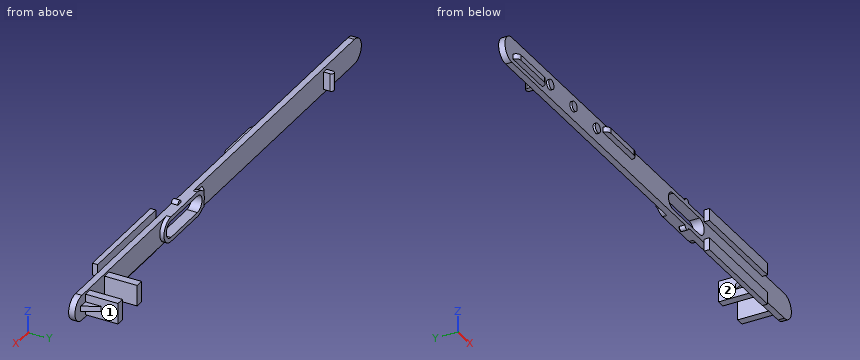
from build123d import *

# Parameters (mm, degrees)
BOSS_EXTRUDE1_DEPTH  = 1.2
BOSS_EXTRUDE2_DEPTH  = 0.8
SKETCH3_W            = 20
SKETCH3_H            = 2.3
BOSS_EXTRUDE3_DEPTH  = 1
SKETCH4_W            = 20
SKETCH4_H            = 2.3
BOSS_EXTRUDE4_DEPTH  = 1
CUT_EXTRUDE1_START   = -0.8
CUT_EXTRUDE1_DEPTH   = 0.8
CUT_EXTRUDE2_START   = -0.8
CUT_EXTRUDE2_DEPTH   = 0.8
CUT_EXTRUDE3_DEPTH   = 50.502424183
BOSS_EXTRUDE5_DEPTH  = 1.2
BOSS_EXTRUDE6_DEPTH  = 1.2
SKETCH10_W           = 1.5
SKETCH10_H           = 4
BOSS_EXTRUDE7_DEPTH  = 6.2
SKETCH11_W           = 1.5
SKETCH11_H           = 4
BOSS_EXTRUDE8_DEPTH  = 6.2
BOSS_EXTRUDE9_DEPTH  = 3.4
BOSS_EXTRUDE10_DEPTH = 1
BOSS_EXTRUDE11_DEPTH = 1
DRAFT1_ANGLE         = 45
SKETCH15_W           = 0.9
SKETCH15_H           = 0.4
SKETCH16_W           = 0.9
SKETCH16_H           = 0.4
SKETCH17_W           = 0.9
SKETCH17_H           = 0.4
RIB1_REACH           = 52.012
SKETCH18_WALL_W      = 105.424996876
SKETCH18_WALL_H      = 1
RIB2_REACH           = 52.012
SKETCH19_WALL_W      = 105.424996876
SKETCH19_WALL_H      = 1
FILLET2_R            = 0.1


with BuildPart() as part:
    # Sketch1 → Boss-Extrude1 (new body)
    with BuildSketch(Plane.XZ):
        with BuildLine():
            Line((46.9, 2.4), (-46.9, 2.4))
            ThreePointArc((-46.9, 2.4), (-49.3, 0), (-46.9, -2.4))
            Line((-46.9, -2.4), (46.9, -2.4))
            ThreePointArc((46.9, -2.4), (49.3, 0), (46.9, 2.4))
        make_face()
    extrude(amount=-BOSS_EXTRUDE1_DEPTH)

    # Sketch2 → Boss-Extrude2 (add)
    with BuildSketch(Plane(origin=(0, 1.2, 0), x_dir=(-1, 0, 0), z_dir=(0, 1, 0))):
        with BuildLine():
            Line((-6.33, 2.4), (-6.33, 0.918))
            Line((-6.33, 0.918), (-6.382506821, 0.918))
            ThreePointArc((-6.382506821, 0.918), (-6.2, 0), (-6.382506821, -0.918))
            Line((-6.382506821, -0.918), (-6.33, -0.918))
            Line((-6.33, -0.918), (-6.33, -2.4))
            Line((-6.33, -2.4), (-17.7, -2.4))
            ThreePointArc((-17.7, -2.4), (-20.1, 0), (-17.7, 2.4))
            Line((-17.7, 2.4), (-6.33, 2.4))
        make_face()
    extrude(amount=BOSS_EXTRUDE2_DEPTH)

    # Sketch3 → Boss-Extrude3 (add)
    with BuildSketch(Plane.XZ):
        with Locations((29.3, 2.85)):
            Rectangle(SKETCH3_W, SKETCH3_H)
    extrude(amount=BOSS_EXTRUDE3_DEPTH)

    # Sketch4 → Boss-Extrude4 (add)
    with BuildSketch(Plane.XZ):
        with Locations((29.3, -2.85)):
            Rectangle(SKETCH4_W, SKETCH4_H)
    extrude(amount=BOSS_EXTRUDE4_DEPTH)

    # Sketch5 → Cut-Extrude1 (cut)
    with BuildSketch(Plane(origin=(0, 2, 0), x_dir=(-1, 0, 0), z_dir=(0, 1, 0)).offset(CUT_EXTRUDE1_START)):
        with BuildLine():
            Line((-8.6, -2.4), (-6.33, -2.4))
            Line((-6.33, -2.4), (-6.33, -1.697))
            Line((-6.33, -1.697), (-6.902887452, -1.697))
            ThreePointArc((-6.902887452, -1.697), (-7.681523, -2.21729565), (-8.6, -2.4))
        make_face()
    extrude(amount=CUT_EXTRUDE1_DEPTH, mode=Mode.SUBTRACT)

    # Sketch6 → Cut-Extrude2 (cut)
    with BuildSketch(Plane(origin=(0, 2, 0), x_dir=(-1, 0, 0), z_dir=(0, 1, 0)).offset(CUT_EXTRUDE2_START)):
        with BuildLine():
            Line((-6.902887452, 1.697), (-6.33, 1.697))
            Line((-6.33, 1.697), (-6.33, 2.4))
            Line((-6.33, 2.4), (-8.6, 2.4))
            ThreePointArc((-8.6, 2.4), (-7.681523, 2.21729565), (-6.902887452, 1.697))
        make_face()
    extrude(amount=CUT_EXTRUDE2_DEPTH, mode=Mode.SUBTRACT)

    # Sketch7 → Cut-Extrude3 (cut, through all)
    with BuildSketch(Plane.XZ):
        with BuildLine():
            Line((17.7, 1.6), (8.6, 1.6))
            ThreePointArc((8.6, 1.6), (7, 0), (8.6, -1.6))
            Line((8.6, -1.6), (17.7, -1.6))
            ThreePointArc((17.7, -1.6), (19.3, 0), (17.7, 1.6))
        make_face()
    extrude(amount=-CUT_EXTRUDE3_DEPTH, mode=Mode.SUBTRACT)

    # Sketch8 → Boss-Extrude5 (add)
    with BuildSketch(Plane.XZ):
        with BuildLine():
            Line((12.7, 2.4), (13.9, 2.4))
            ThreePointArc((13.9, 2.4), (13.3, 3), (12.7, 2.4))
        make_face()
    extrude(amount=-BOSS_EXTRUDE5_DEPTH)

    # Sketch9 → Boss-Extrude6 (add)
    with BuildSketch(Plane.XZ):
        with BuildLine():
            Line((13.9, -2.4), (12.7, -2.4))
            ThreePointArc((12.7, -2.4), (13.3, -3), (13.9, -2.4))
        make_face()
    extrude(amount=-BOSS_EXTRUDE6_DEPTH)

    # Sketch10 → Boss-Extrude7 (add)
    with BuildSketch(Plane(origin=(0, 1.2, 0), x_dir=(-1, 0, 0), z_dir=(0, 1, 0))):
        with Locations((-38.35, 0)):
            Rectangle(SKETCH10_W, SKETCH10_H)
    extrude(amount=BOSS_EXTRUDE7_DEPTH)

    # Sketch11 → Boss-Extrude8 (add)
    with BuildSketch(Plane(origin=(0, 1.2, 0), x_dir=(-1, 0, 0), z_dir=(0, 1, 0))):
        with Locations((-44.95, 0)):
            Rectangle(SKETCH11_W, SKETCH11_H)
    extrude(amount=BOSS_EXTRUDE8_DEPTH)

    # Sketch12 → Boss-Extrude9 (add)
    with BuildSketch(Plane(origin=(0, 0, -1.7), x_dir=(-1, 0, 0), z_dir=(0, 0, -1))):
        with BuildLine():
            Line((36.3, 1.2), (37.3, 1.2))
            Line((37.3, 1.2), (37.3, 2.4))
            ThreePointArc((37.3, 2.4), (36.8, 2.9), (36.3, 2.4))
            Line((36.3, 2.4), (36.3, 1.2))
        make_face()
    extrude(amount=-BOSS_EXTRUDE9_DEPTH)

    # Sketch13 → Boss-Extrude10 (add)
    with BuildSketch(Plane(origin=(0, 0, -1.6), x_dir=(-1, 0, 0), z_dir=(0, 0, -1))):
        with BuildLine():
            Line((46.5, 0), (36.5, 0))
            ThreePointArc((36.5, 0), (36.792893219, -0.707106781), (37.5, -1))
            Line((37.5, -1), (45.5, -1))
            ThreePointArc((45.5, -1), (46.207106781, -0.707106781), (46.5, 0))
        make_face()
    extrude(amount=-BOSS_EXTRUDE10_DEPTH)

    # Sketch14 → Boss-Extrude11 (add)
    with BuildSketch(Plane(origin=(0, 0, 0.6), x_dir=(-1, 0, 0), z_dir=(0, 0, -1))):
        with BuildLine():
            Line((15.6, 0), (5.6, 0))
            ThreePointArc((5.6, 0), (5.892893219, -0.707106781), (6.6, -1))
            Line((6.6, -1), (14.6, -1))
            ThreePointArc((14.6, -1), (15.307106781, -0.707106781), (15.6, 0))
        make_face()
    extrude(amount=-BOSS_EXTRUDE11_DEPTH)

    # Draft1
    draft1_faces = [part.faces().sort_by_distance(p)[0] for p in [
        (6.33, 1.6, -1.3075),
        (6.33, 1.6, 1.3075),
    ]]
    draft(draft1_faces, Plane(origin=(8.6, 2, 0), x_dir=(1, 0, 0), z_dir=(0, 1, 0)), DRAFT1_ANGLE)

    # Sketch15 → Revolve1 (revolve)
    with BuildSketch(Plane(origin=(0, 0, 0), x_dir=(-1, 0, 0), z_dir=(0, 0, -1)), mode=Mode.PRIVATE) as revolve1_sk:
        with Locations((25.6, -0.2)):
            Rectangle(SKETCH15_W, SKETCH15_H)
    revolve(revolve1_sk.sketch.rotate(Axis((-26.05, -0.4, 0), (0, 1, 0)), 270), axis=Axis((-26.05, -0.4, 0), (0, 1, 0)))

    # Sketch16 → Revolve2 (revolve)
    with BuildSketch(Plane(origin=(0, 0, 0), x_dir=(-1, 0, 0), z_dir=(0, 0, -1)), mode=Mode.PRIVATE) as revolve2_sk:
        with Locations((33.6, -0.2)):
            Rectangle(SKETCH16_W, SKETCH16_H)
    revolve(revolve2_sk.sketch.rotate(Axis((-34.05, -0.4, 0), (0, 1, 0)), 270), axis=Axis((-34.05, -0.4, 0), (0, 1, 0)))

    # Sketch17 → Revolve3 (revolve)
    with BuildSketch(Plane(origin=(0, 0, 0), x_dir=(-1, 0, 0), z_dir=(0, 0, -1)), mode=Mode.PRIVATE) as revolve3_sk:
        with Locations((17.6, -0.2)):
            Rectangle(SKETCH17_W, SKETCH17_H)
    revolve(revolve3_sk.sketch.rotate(Axis((-18.05, -0.4, 0), (0, 1, 0)), 270), axis=Axis((-18.05, -0.4, 0), (0, 1, 0)))

    # Sketch18 wall → Rib1 (add, up to next)
    with BuildSketch(Plane(origin=(46.5, 2.7, 0), x_dir=(0.470588235294, -0.882352941176, 0), z_dir=(-0.882352941176, -0.470588235294, 0)), mode=Mode.PRIVATE) as rib1_sk1:
        Rectangle(SKETCH18_WALL_W, SKETCH18_WALL_H)
    rib1_tool1 = extrude(rib1_sk1.sketch, amount=RIB1_REACH, mode=Mode.PRIVATE) - part.part
    add(rib1_tool1.solids().sort_by_distance((46.5, 2.7, 0))[0])

    # Sketch19 wall → Rib2 (add, up to next)
    with BuildSketch(Plane(origin=(36.8, 2.7, 0), x_dir=(-0.470588235294, -0.882352941176, 0), z_dir=(0.882352941176, -0.470588235294, 0)), mode=Mode.PRIVATE) as rib2_sk1:
        Rectangle(SKETCH19_WALL_W, SKETCH19_WALL_H)
    rib2_tool1 = extrude(rib2_sk1.sketch, amount=RIB2_REACH, mode=Mode.PRIVATE) - part.part
    add(rib2_tool1.solids().sort_by_distance((36.8, 2.7, 0))[0])

    # Fillet2
    fillet2_edges = [part.edges().sort_by_distance(p)[0] for p in [
        (13.3, 1.2, -3),
    ]]
    fillet(fillet2_edges, radius=FILLET2_R)


solid = part.part
Build history of the part. All positions in model axes, mm. Face numbers are marked on the shaded views. Give positions to 0.01 mm unless a question says otherwise; leave off trailing zeros. Order: outer loops, then holes, each group sorted by start corner. A loop starts at its lowest first (then second) coordinate and runs counter-clockwise, first axis right, second up. Notation, with made-up numbers: M 32.25,4.5 L 37.25,4.5 A13 ccw 37.25,16.5 Z; hole C 68.5,-3 d4. An arc over 180 degrees is marked long. Put each result on its own line as item: value.
Item 1: Slice it at B-B, the plane x = 29. Write the cut outline in (y, z), plus the area to 3 significant figures.
From the geometry:
outline: M -1,-4 L 0,-4 L 0,-2.4 L 1.2,-2.4 L 1.2,2.4 L 0,2.4 L 0,4 L -1,4 L -1,1.7 L 0,1.7 L 0,-1.7 L -1,-1.7 Z
area: 10.4 mm2
Item 2: Probe line 1 (X direction, y = 2.25, z = -1); line 2 (X direction, y = 4, z = 1); line 3 (Y direction, x = 24.5, z = 0). List the from-to ranges inside material, lowest first. Write a range as [from, to].
From the geometry:
line 1: x = [-37.3, -36.3], [37.6, 39.1], [44.2, 45.7]
line 2: x = [37.6, 39.1], [44.2, 45.7]
line 3: y = [0, 1.2]
Item 3: Slice it at A-A, the plane y = 6. Write the cut outline in (x, z).
From the geometry:
outline: M 37.6,-2 L 39.1,-2 L 39.1,2 L 37.6,2 Z; M 44.2,-2 L 45.7,-2 L 45.7,2 L 44.2,2 Z
Item 4: Two-plate mould, pull along X, no slides. Class the marked faces 1 and 2: +X half, -X half, draft (parallel to the pull), parting line (faces both ways), or undercut.
From the geometry:
face 1: +X half
face 2: undercut
Item 5: Flat gauge pins, fed straight in: pin 1 Ø1.3 at (x, y) = (46.5, 2.5) entering from -Z; pin 2 Ø2 at (y, z) = (5.5, -1) entering from -X; pin 3 Ø4 at (y, z) = (0.5, 3) entering from +X. Where does each tip first touch, or does it go through?
From the geometry:
pin 1: stops at z = -0.5
pin 2: stops at x = 37.6
pin 3: stops at x = 49.08
